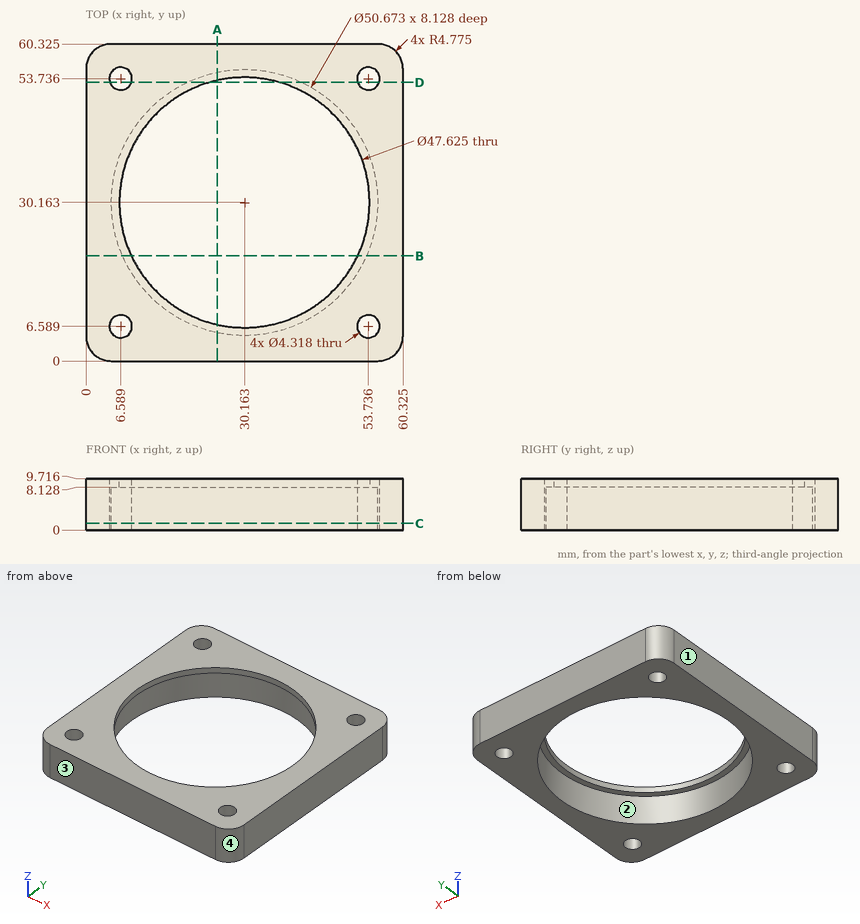
Could you check a few things on this drawing? It's one solid part, dimensions in mm from its lowest x, y, z. Give positions to 0.01 mm unless a question says otherwise; leave off trailing zeros. Write each loop counter-clockwise with the first axis right and the second up, starting at its lowest first coordinate (ties: lowest second). Pieces come first, ordered by that corner, then holes. Notation, with made-up numbers: M -16.75,46 L 9.25,46 A16 ccw 9.25,77 Z; hole C -10.5,-33 d1. An arc over 180 degrees is marked long. Put each result on its own line as item: value. Start each with the question number.
Item 1: If we section it at B-B, the plane y = 20: Write out the boundary of the cut face in (x, z) (1 decimal).
Item 2: I need wall thicknesses on L1, parallel to Y at x = 8.5, z = 5.5 (1 decimal); L2, parallel to Y at x = 31, z = 1.75 (1 decimal); L3, parallel to Z at x = 5, y = 31.5 (1 decimal). Which ranges of each line are inside material? Lowest first, please. Write a range as from..to.
Item 3: If we section it at C-C, the plane z = 1.25: Count the separate pieces of the cut face and the enclosed holes in it, then the cut area to 3 significant figures.
Item 4: Thinking about a two-plate mould opening in X: for the marked faces 1, 2, 3 and 4, which applies, +X half, -X half, draft (parallel to the pull), parting line (faces both ways), or undercut?
Item 5: If we section it at D-D, the plane y = 53: Write out the boundary of the cut face in (x, z) (1 decimal).
Item 6: If we section it at A-A, the plane x = 25: Write out the boundary of the cut face in (y, z) (1 decimal).
Values:
1. outline: M 0,0 L 7,0 L 7,8.1 L 8.6,8.1 L 8.6,9.7 L 0,9.7 Z; M 51.7,8.1 L 53.4,8.1 L 53.4,0 L 60.3,0 L 60.3,9.7 L 51.7,9.7 Z
2. L1: 0..5.6, 7.6..17, 43.3..52.7, 54.7..60.3
2. L2: 0..4.8, 55.5..60.3
2. L3: 8.1..9.7
3. separate pieces: 1
3. enclosed holes: 5
3. area: 1,540 mm²
4. face 1: -X half
4. face 2: undercut
4. face 3: draft
4. face 4: +X half
5. outline: M 0,0 L 4.6,0 L 4.6,9.7 L 0,9.7 Z; M 8.6,0 L 19.2,0 L 19.2,8.1 L 23.4,8.1 L 23.4,9.7 L 8.6,9.7 Z; M 36.9,8.1 L 41.1,8.1 L 41.1,0 L 51.7,0 L 51.7,9.7 L 36.9,9.7 Z; M 55.8,0 L 60.3,0 L 60.3,9.7 L 55.8,9.7 Z
6. outline: M 0,0 L 5.4,0 L 5.4,8.1 L 6.9,8.1 L 6.9,9.7 L 0,9.7 Z; M 53.4,8.1 L 55,8.1 L 55,0 L 60.3,0 L 60.3,9.7 L 53.4,9.7 Z
